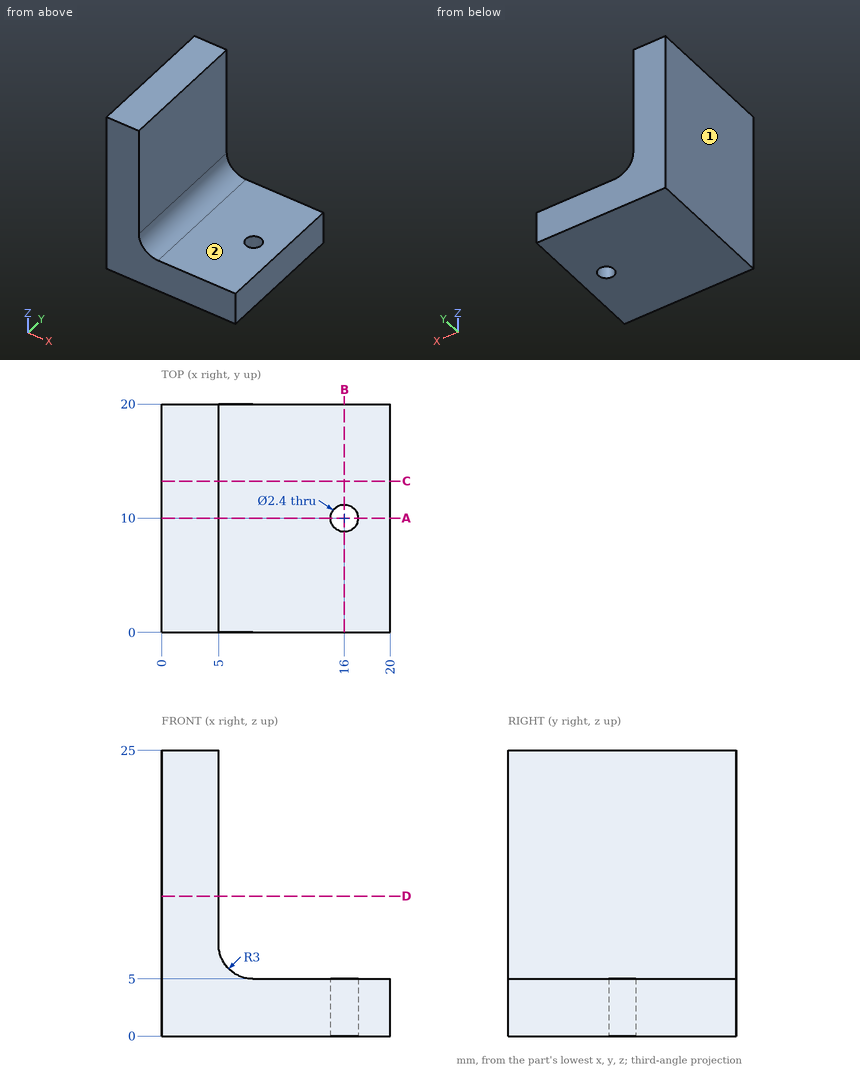
Design review of the part shown in the three views and the two pictorial views. Dimensions are in mm from the part's minimum x, y and z. A direction names the side the tool comes from. Round coordinates to 2 decimals unless told otherwise and drop trailing zeros. Write each loop counter-clockwise with the first axis right and the second up, starting at its lowest first coordinate (ties: lowest second). Pieces come first, ordered by that corner, then holes. Notation, with made-up numbers: (87.25, 53) - (113.25, 53) arc R34 ccw to (113.25, 85) - close; hole circle Ø8 at (-18, 59). An arc over 180 degrees is marked (long way). Answer as CSV lines item,"result". Start each with the question number.
(1) For pin 1 (10 mm diameter, centred on y = 15, z = 8, fed in from -X); pin 2 (9.5 mm diameter, centred on x = 13, y = 8, fed in from +Z); pin 3 (6 mm diameter, centred on y = 7, z = 11, fed in from +X); pin 4 (2 mm diameter, centred on x = 16, y = 10, fed in from -Z), all flat-tipped, find the tip position at first contact; note any pin that passes through.
(2) Add section D-D, the plane z = 12.25. State the section outline as (x, y) points, plus the area to 3 significant figures.
(3) For line 1 (Y direction, x = 16, z = 2.3); line 2 (Z direction, x = 11.75, y = 16.5), list the stretches that pass through material, from the lowest coordinate up.
(4) Add section B-B, the plane x = 16. State the section outline as (y, z) points.
(5) Machinability: for the marked faces 1 and 2, which of the approach directions +Z, -Z, +X, -X, +Y, -Y give a long, thin tool a straight path to every point of the face, cutting with its end or side? Answer none if there is none.
(6) Add section C-C, the plane y = 13.25. State the section outline as (x, z) points.
(7) Add section A-A, the plane y = 10. State the section outline as (x, z) points, plus the area to 3 significant figures.
From the geometry:
1,pin 1,"stops at x = 0"
1,pin 2,"stops at z = 5"
1,pin 3,"stops at x = 5"
1,pin 4,"passes through"
2,outline,"(0, 0) - (5, 0) - (5, 20) - (0, 20) - close"
2,area,"100 mm²"
3,line 1,"y = 0 to 8.8, 11.2 to 20"
3,line 2,"z = 0 to 5"
4,outline,"(0, 0) - (8.8, 0) - (8.8, 5) - (0, 5) - close; (11.2, 0) - (20, 0) - (20, 5) - (11.2, 5) - close"
5,face 1,"+Z, -Z, -X, +Y, -Y"
5,face 2,"+Z, +X, +Y, -Y"
6,outline,"(0, 0) - (20, 0) - (20, 5) - (8, 5) arc R3 cw to (5, 8) - (5, 25) - (0, 25) - close"
7,outline,"(0, 0) - (14.8, 0) - (14.8, 5) - (8, 5) arc R3 cw to (5, 8) - (5, 25) - (0, 25) - close; (17.2, 0) - (20, 0) - (20, 5) - (17.2, 5) - close"
7,area,"190 mm²"
